```python
from build123d import *

# Parameters (mm, degrees)
SKETCH1_W           = 51.5
SKETCH1_H           = 80
SKETCH1_R           = 1.65
SKETCH1_R_2         = 1.375
SKETCH1_W_2         = 12
SKETCH1_H_2         = 6
BOSS_EXTRUDE1_DEPTH = 6.25


with BuildPart() as part:
    # Sketch1 → Boss-Extrude1 (new body)
    with BuildSketch(Plane(origin=(0, 0, 0), x_dir=(1, 0, 0), z_dir=(0, 1, 0))):
        with Locations((25.75, 40)):
            Rectangle(SKETCH1_W, SKETCH1_H)
        with Locations(Location((10.75, 15, 0), (0, 0, 270))):
            Circle(SKETCH1_R, mode=Mode.SUBTRACT)
        with Locations(Location((40.75, 15, 0), (0, 0, 270))):
            Circle(SKETCH1_R, mode=Mode.SUBTRACT)
        with Locations(Location((25.75, 73.95, 0), (0, 0, 270))):
            Circle(SKETCH1_R_2, mode=Mode.SUBTRACT)
        with Locations(Location((40.75, 40, 0), (0, 0, 270))):
            Circle(SKETCH1_R, mode=Mode.SUBTRACT)
        with Locations(Location((25.75, 6.05, 0), (0, 0, 270))):
            Circle(SKETCH1_R_2, mode=Mode.SUBTRACT)
        with Locations(Location((40.75, 65, 0), (0, 0, 270))):
            Circle(SKETCH1_R, mode=Mode.SUBTRACT)
        with Locations(Location((10.75, 40, 0), (0, 0, 270))):
            Circle(SKETCH1_R, mode=Mode.SUBTRACT)
        with Locations(Location((10.75, 65, 0), (0, 0, 270))):
            Circle(SKETCH1_R, mode=Mode.SUBTRACT)
        with Locations((41.875, 73.95)):
            Rectangle(SKETCH1_W_2, SKETCH1_H_2, mode=Mode.SUBTRACT)
        with Locations((41.875, 6.05)):
            Rectangle(SKETCH1_W_2, SKETCH1_H_2, mode=Mode.SUBTRACT)
        with Locations((9.625, 6.05)):
            Rectangle(SKETCH1_W_2, SKETCH1_H_2, mode=Mode.SUBTRACT)
        with Locations((9.625, 73.95)):
            Rectangle(SKETCH1_W_2, SKETCH1_H_2, mode=Mode.SUBTRACT)
    extrude(amount=BOSS_EXTRUDE1_DEPTH)


solid = part.part
```
Geometry: final body of the model. Coordinates: model frame, mm. A direction names the side the tool comes from. Round coordinates to 2 decimals unless told otherwise and drop trailing zeros. Order: outer loops, then holes, each group sorted by start corner. A loop starts at its lowest first (then second) coordinate and runs counter-clockwise, first axis right, second up. Notation, with made-up numbers: (59, 13) - (81, 13) arc R23 ccw to (81, 31) - close; hole circle Ø6 at (74, 37). An arc over 180 degrees is marked (long way). Write item = value, one per line. Start each with the question number.
Q1. Access query for faces 1 (the flat face through (10, 3, -70.95)), 2 (the flat face through (25, 6.25, -41)). Directions: +Z, -Z, +X, -X, +Y, -Y. A direction counts if a zero-diameter tool reaches every point of the face in a straight line with its end or side. Return the directions, or none.
Q2. Pull-direction query (X, two-part tool) for faces 3 (the flat face through (0, 3, -39)), 4 (the flat face through (25, 3, 0)), 5 (the cylindrical face through (10.82, 3.08, -66.65)); classes: +X half, -X half, draft (parallel to the pull), parting line (faces both ways), or undercut.
Q3. Cut plane D-D on z = -40. Return the cut outline in (x, y), and give its area (3 significant figures).
Q4. Ray query, line 1 (X direction, y = 2.75, z = -40); line 2 (Z direction, x = 43.5, y = 2.75); line 3 (X direction, y = 2.5, z = -73.95) (3 decimals). Return the intervals inside material, ascending. Write a range as from..to.
Q5. Cut plane C-C on z = -6.05. Return the cut outline in (x, y) (3 decimals).
Q6. Cut plane B-B on x = 10.75. Return the cut outline in (y, z), and give its area (3 significant figures).
Q7. Pin query (flat end, axial travel): pin 1 (1.6 mm diameter, centred on x = 25.75, z = -73.95, fed in from +Y). Return the tip coordinate at first contact, or that it passes through.
Q8. Cut plane A-A on y = 2. Give the number of separate pieces and of enclosed holes in the cut face, and give its area (3 significant figures).
Outcome:
q1.face_1 = +Y, -Y
q1.face_2 = +Z, -Z, +X, -X, +Y
q2.face_3 = -X half
q2.face_4 = draft
q2.face_5 = undercut
q3.outline = (0, 0) - (9.1, 0) - (9.1, 6.25) - (0, 6.25) - close; (12.4, 0) - (39.1, 0) - (39.1, 6.25) - (12.4, 6.25) - close; (42.4, 0) - (51.5, 0) - (51.5, 6.25) - (42.4, 6.25) - close
q3.area = 281 mm^2
q4.line_1 = 0..9.1, 12.4..39.1, 42.4..51.5
q4.line_2 = -80..-76.95, -70.95..-9.05, -3.05..0
q4.line_3 = 0..3.625, 15.625..24.375, 27.125..35.875, 47.875..51.5
q5.outline = (0, 0) - (3.625, 0) - (3.625, 6.25) - (0, 6.25) - close; (15.625, 0) - (24.375, 0) - (24.375, 6.25) - (15.625, 6.25) - close; (27.125, 0) - (35.875, 0) - (35.875, 6.25) - (27.125, 6.25) - close; (47.875, 0) - (51.5, 0) - (51.5, 6.25) - (47.875, 6.25) - close
q6.outline = (0, -80) - (6.25, -80) - (6.25, -76.95) - (0, -76.95) - close; (0, -70.95) - (6.25, -70.95) - (6.25, -66.65) - (0, -66.65) - close; (0, -63.35) - (6.25, -63.35) - (6.25, -41.65) - (0, -41.65) - close; (0, -38.35) - (6.25, -38.35) - (6.25, -16.65) - (0, -16.65) - close; (0, -13.35) - (6.25, -13.35) - (6.25, -9.05) - (0, -9.05) - close; (0, -3.05) - (6.25, -3.05) - (6.25, 0) - (0, 0) - close
q6.area = 363 mm^2
q7.pin_1 = through
q8.separate_pieces = 1
q8.enclosed_holes = 12
q8.area = 3,770 mm^2
